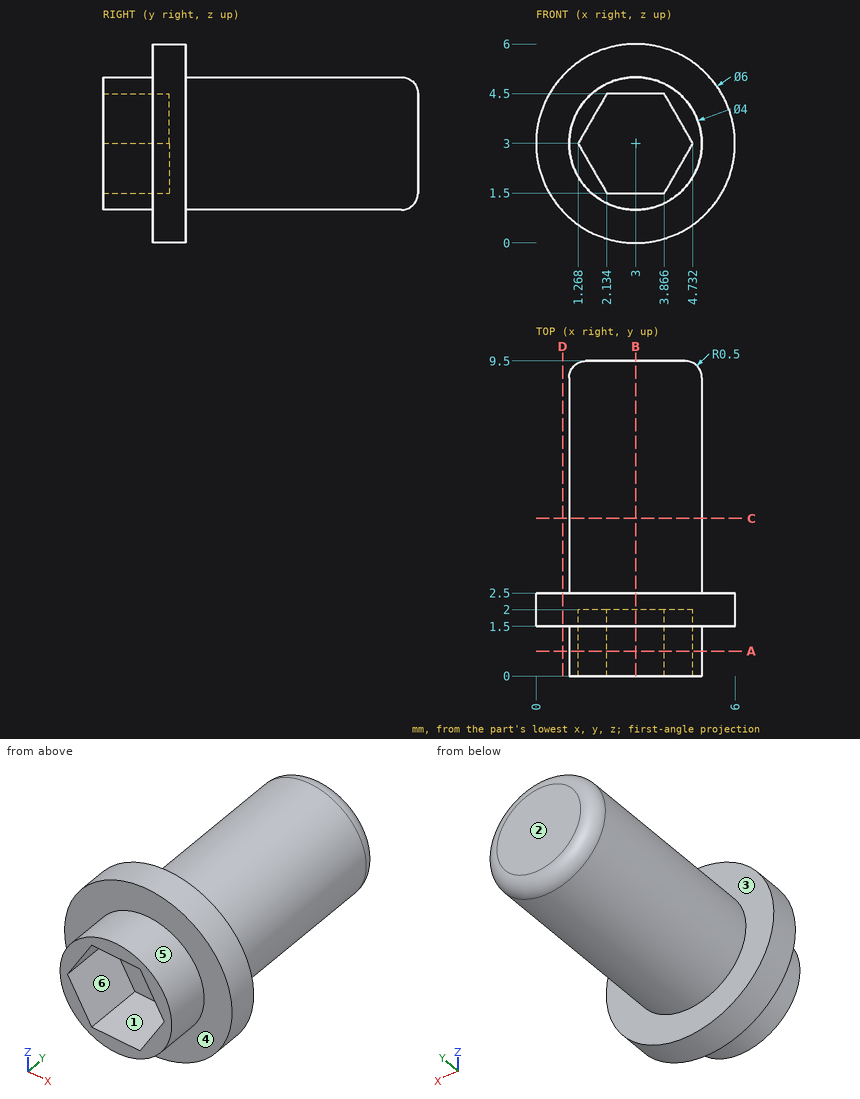
Print and shaded views of the part. All mm, measured from the part's lowest x, y and z. A direction names the side the tool comes from. Give positions to 0.01 mm unless a question says otherwise; leave off trailing zeros. Loops run counter-clockwise (first coordinate to the right, second up) from the corner with the lowest first, then second, coordinate; pieces in that order, holes last. Notation, with made-up numbers: M 13,55 L 47,55 A26 ccw 47,79 Z; hole C -16.5,5 d3. An arc over 180 degrees is marked long. Write each question's results on one line, items separated by ' | '.
Q1. Which spindle directions (+Z, -Z, +X, -X, +Y, -Y) get a long thin tool onto all of the face, cutting with end or side? Do the marked faces 1, 2 and 3. Say none if no direction does.
Geometry check:
face 1: -Y | face 2: +Z, -Z, +X, -X, +Y | face 3: +Y
Q2. Band-saw the part on C-C on y = 4.75. Write the cut outline in (x, z).
Geometry check:
outline: C 3,3 d4
Q3. Band-saw the part on D-D on x = 0.8. Write the cut outline in (y, z), and give its area (3 significant figures).
Geometry check:
outline: M 1.5,0.96 L 2.5,0.96 L 2.5,5.04 L 1.5,5.04 Z | area: 4.08 mm²
Q4. Band-saw the part on A-A on y = 0.75. Write the cut outline in (x, z), and give its area (3 significant figures).
Geometry check:
outline: C 3,3 d4; hole M 1.27,3 L 2.13,1.5 L 3.87,1.5 L 4.73,3 L 3.87,4.5 L 2.13,4.5 Z | area: 4.77 mm²
Q5. Flat gauge pins, fed straight in: P1, Ø0.9, axis at x = 2.5, z = 3, coming from the -Y side; P2, Ø1.5, axis at y = 5.5, z = 3, coming from the -X side; P3, Ø1.9, axis at x = 3, y = 0.5, coming from the +Z side. Where does each tip first touch, or does it go through?
Geometry check:
P1: stops at y = 2 | P2: stops at x = 1 | P3: stops at z = 5
Q6. Band-saw the part on B-B on x = 3. Write the cut outline in (y, z), and give its area (3 significant figures).
Geometry check:
outline: M 0,1 L 1.5,1 L 1.5,0 L 2.5,0 L 2.5,1 L 9,1 A0.5 ccw 9.5,1.5 L 9.5,4.5 A0.5 ccw 9,5 L 2.5,5 L 2.5,6 L 1.5,6 L 1.5,5 L 0,5 L 0,4.5 L 2,4.5 L 2,1.5 L 0,1.5 Z | area: 33.9 mm²
Q7. Probe probe 1 along Y at (x, z) = (3.75, 5.3); probe 2 along Z at (x, y) = (3.2, 0.75); probe 3 along Y at (x, z) = (2, 2.75). List the from-to ranges inside material, lowest first.
Geometry check:
probe 1: y = 1.5 to 2.5 | probe 2: z = 1.01 to 1.5, 4.5 to 4.99 | probe 3: y = 2 to 9.5
Q8. Mould opens along X. For the marked faces 4, 5 and 6 say: pulls with the +X half, pulls with the -X half, needs draft (parallel to the pull), parting line crosses it, or undercut.
Geometry check:
face 4: needs draft | face 5: parting line crosses it | face 6: undercut
